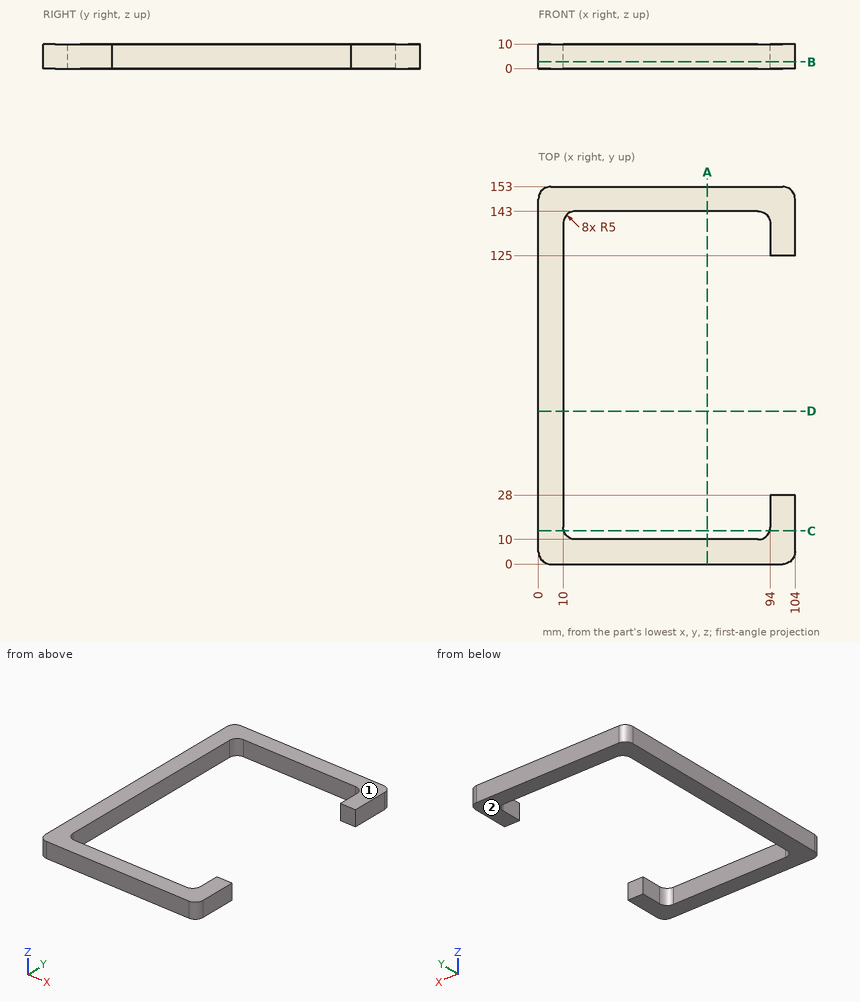
Answer from the drawing. Dimensions are ordinates in mm from the lowest x, y and z of the part. Give positions to 0.01 mm unless a question says otherwise; leave off trailing zeros. Write each loop counter-clockwise with the first axis right and the second up, starting at its lowest first coordinate (ties: lowest second). Pieces come first, ordered by that corner, then holes. Notation, with made-up numbers: (15, 52.25) -> (66, 52.25) arc R21 cw to (66, 69.25) -> close; hole circle Ø2 at (-25, 15.25). An arc over 180 degrees is marked (long way). One line per question, with ' | ' between items. Start each with the question number.
1. Section A-A (x = 68.5) is taken. Determine the outline of the cut face in (y, z), plus the area to 3 significant figures.
2. Find the intervals of material crossed by probe 1 along Y at (x, z) = (40, 1.5); probe 2 along X at (y, z) = (126, 4.5); probe 3 along X at (y, z) = (43.5, 5), in increasing order.
3. For a pull along Z with two mould halves and no side action, classify the marked faces 1 and 2 as pulls with the +Z half, pulls with the -Z half, needs draft (parallel to the pull), parting line crosses it, or undercut.
4. Section D-D (y = 62) is taken. Determine the outline of the cut face in (x, z).
5. Given pin 1 Ø3 at (y, z) = (72, 4) entering from +X, flat-ended and moving along its own axis, determine where the tip first touches the part or whether it passes through.
6. Section C-C (y = 13.5) is taken. Determine the outline of the cut face in (x, z).
7. Section B-B (z = 2.75) is taken. Determine the outline of the cut face in (x, y).
Response values:
1) outline: (0, 0) -> (10, 0) -> (10, 10) -> (0, 10) -> close; (143, 0) -> (153, 0) -> (153, 10) -> (143, 10) -> close | area: 200 mm2
2) probe 1: 0 to 10, 143 to 153 | probe 2: 0 to 10, 94 to 104 | probe 3: 0 to 10
3) face 1: pulls with the +Z half | face 2: pulls with the -Z half
4) outline: (0, 0) -> (10, 0) -> (10, 10) -> (0, 10) -> close
5) pin 1: x = 10
6) outline: (0, 0) -> (10.23, 0) -> (10.23, 10) -> (0, 10) -> close; (93.77, 0) -> (104, 0) -> (104, 10) -> (93.77, 10) -> close
7) outline: (0, 5) arc R5 ccw to (5, 0) -> (99, 0) arc R5 ccw to (104, 5) -> (104, 28) -> (94, 28) -> (94, 15) arc R5 cw to (89, 10) -> (15, 10) arc R5 cw to (10, 15) -> (10, 138) arc R5 cw to (15, 143) -> (89, 143) arc R5 cw to (94, 138) -> (94, 125) -> (104, 125) -> (104, 148) arc R5 ccw to (99, 153) -> (5, 153) arc R5 ccw to (0, 148) -> close
